Answer from the drawing. Dimensions are ordinates in mm from the lowest x, y and z of the part. Give positions to 0.01 mm unless a question says otherwise; leave off trailing zeros. Order: outer loops, then holes, each group sorted by start corner. A loop starts at its lowest first (then second) coordinate and runs counter-clockwise, first axis right, second up. Notation, with made-up numbers: (37, -6) -> (57, -6) arc R26 ccw to (57, 20) -> close; hole circle Ø6 at (-18, -10.75). An arc over 180 degrees is marked (long way). Answer as CSV lines item,"result". Start each with the question number.
1) Find section B-B (y = 19.05). Determine the outline of the cut face in (x, z), and give its area (3 significant figures).
2) Flat-ended cylindrical pins translate along their axes: pin 1 Ø10 at (x, y) = (79, 12.5) entering from +Z; pin 2 Ø3 at (x, y) = (70.5, 20) entering from +Z. Find the tip coordinate at first contact, or state that the pin passes through.
3) Find section D-D (y = 28). Determine the outline of the cut face in (x, z) (1 decimal).
4) Straight lines are drawn through the part: L1, parallel to X at y = 21, z = 0.2; L2, parallel to Y at x = 82.55, z = 1.75; L3, parallel to Y at x = 5, z = 3.95. For each, find the intervals that lie inside material, in ascending order. Write a range as from..to.
5) Find section A-A (x = 82.55). Determine the outline of the cut face in (y, z).
6) Find section C-C (z = 1.5). Determine the outline of the cut face in (x, y).
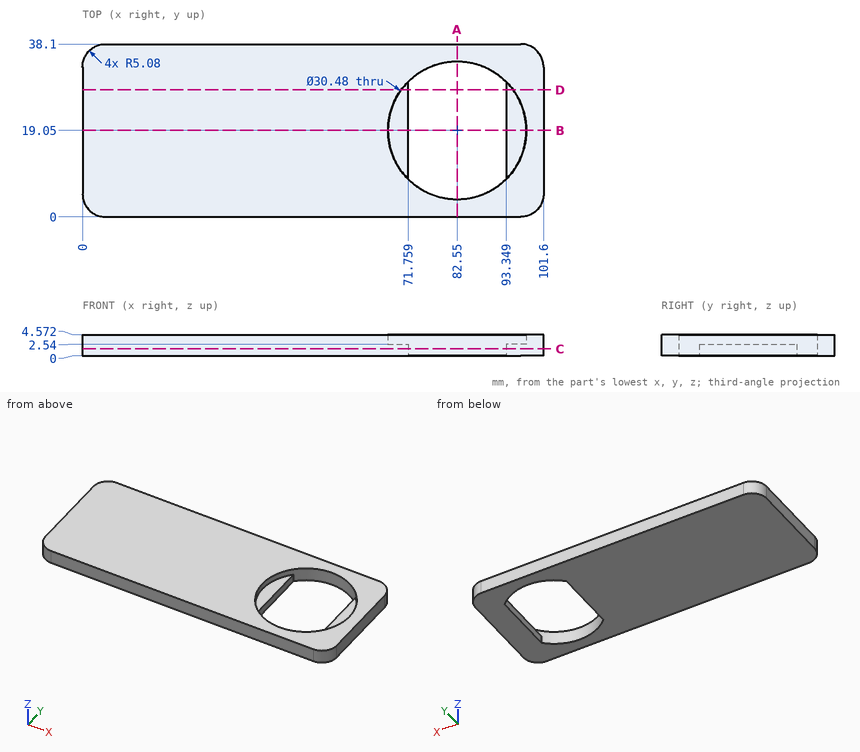
Findings below:
1,outline,"(0, 0) -> (71.76, 0) -> (71.76, 2.54) -> (67.31, 2.54) -> (67.31, 4.57) -> (0, 4.57) -> close; (93.35, 0) -> (101.6, 0) -> (101.6, 4.57) -> (97.79, 4.57) -> (97.79, 2.54) -> (93.35, 2.54) -> close"
1,area,"348 mm²"
2,pin 1,"through"
2,pin 2,"z = 2.54"
3,outline,"(0, 0) -> (71.8, 0) -> (71.8, 2.5) -> (70.2, 2.5) -> (70.2, 4.6) -> (0, 4.6) -> close; (93.3, 0) -> (101.6, 0) -> (101.6, 4.6) -> (94.9, 4.6) -> (94.9, 2.5) -> (93.3, 2.5) -> close"
4,L1,"0..71.76, 93.35..101.6"
4,L2,"0..3.81, 34.29..38.1"
4,L3,"0..38.1"
5,outline,"(0, 0) -> (3.81, 0) -> (3.81, 4.57) -> (0, 4.57) -> close; (34.29, 0) -> (38.1, 0) -> (38.1, 4.57) -> (34.29, 4.57) -> close"
6,outline,"(0, 5.08) arc R5.08 ccw to (5.08, 0) -> (96.52, 0) arc R5.08 ccw to (101.6, 5.08) -> (101.6, 33.02) arc R5.08 ccw to (96.52, 38.1) -> (5.08, 38.1) arc R5.08 ccw to (0, 33.02) -> close; hole (71.76, 8.29) arc R15.24 ccw to (93.35, 8.3) -> (93.35, 29.8) arc R15.24 ccw to (71.76, 29.81) -> close"
